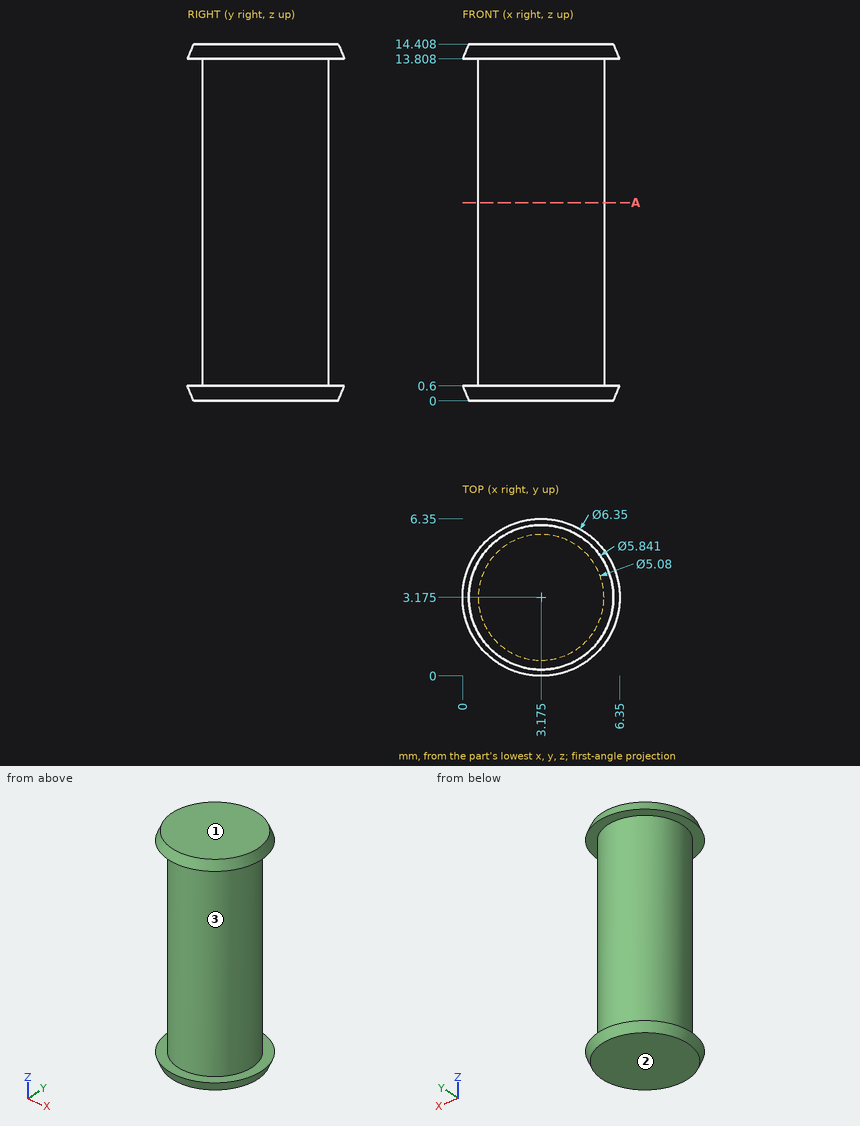
Study the drawing (mm; zero at the part's minimum x, y, z) and answer. Coordinates: 2 decimals unless noted, no trailing zeros. Write each loop counter-clockwise with the first axis right and the second up, starting at its lowest first coordinate (ties: lowest second). Pieces come first, ordered by that corner, then holes.
Q1. Given P1, Ø3, axis at x = 1.5, z = 12, coming from the -Y side, flat-ended and moving along its own axis, determine where the tip first touches the part or whether it passes through.
Returned:
P1: stops at y = 0.64
Q2. Find the intervals of material crossed by line 1 along Z through (x, y) = (3.25, 0.5); line 2 along Y through (x, z) = (3.75, 4.5); line 3 along Y through (x, z) = (1.5, 9.5) (1 decimal), in increasing order.
Returned:
line 1: z = 0 to 0.6, 13.81 to 14.41
line 2: y = 0.7 to 5.65
line 3: y = 1.3 to 5.1
Q3. The mould has two halves that part along Z. Classify the marked faces 1, 2 and 3: released by +Z, released by -Z, zero draft, split by the parting line, or undercut.
Returned:
face 1: released by +Z
face 2: released by -Z
face 3: undercut
Q4. Section A-A, the plane z = 8 is taken. Write down the section's boundary in (x, y) (1 decimal).
Returned:
outline: circle Ø5.1 at (3.2, 3.2)
